Source: CAD feature listing. Evaluate the final solid. Frame: model axes, mm. Face numbers are marked on the shaded views. A direction names the side the tool comes from. Coordinates: 2 decimals unless noted, no trailing zeros. Write each loop counter-clockwise with the first axis right and the second up, starting at its lowest first coordinate (ties: lowest second). Pieces come first, ordered by that corner, then holes. Notation, with made-up numbers: M 71,4 L 100,4 A16 ccw 100,20 Z; hole C -1,0 d11. An arc over 180 degrees is marked long. One line per item, written item: value. Start each with the question number.
Item 1: Cut plane D-D, the plane z = 3.25. State how many separate pieces and enclosed holes the cut face has, then the cut area to 3 significant figures.
Item 2: Pin query (flat end, axial travel): P1, Ø3.5, axis at x = 14, y = 15, coming from the +Z side; P2, Ø2.5, axis at x = -1, z = 3.5, coming from the +Y side. Return the tip coordinate at first contact, or that it passes through.
Item 3: Cut plane A-A, the plane y = -26.5. Output: boundary loops of the cut face in (x, z).
Item 4: Cut plane B-B, the plane x = 10. Output: boundary loops of the cut face in (y, z).
Item 5: Mould query, pull axis X, two halves, no side actions, for the marked faces 1, 2 and 3. Classes: released by +X, released by -X, zero draft, split by the parting line, or undercut.
Item 6: Cut plane C-C, the plane x = -1. Output: boundary loops of the cut face in (y, z), then the cut area to 3 significant figures.
Item 7: Set-up query: the marked faces 4, 5 and 6. Return all of +Z, -Z, +X, -X, +Y, -Y with unobstructed straight access to the full face (end or side cutting, diameter ignored); none if empty.
Item 8: Ray query, L1, parallel to Y at x = 2, z = 2.25; L2, parallel to Y at x = -6, z = 2.1; L3, parallel to X at y = 6, z = 1.6. Return the intervals inside material, ascending. Write a range as from..to.
```python
from build123d import *

# Parameters (mm, degrees)
SKETCH_1_W          = 35
SKETCH_1_H          = 60
EXTRUDE_1_DEPTH     = 5
SKETCH_2_R          = 1.5
SKETCH_2_R_2        = 0.5
SKETCH_2_W          = 15
SKETCH_2_H          = 10
CUT_EXTRUDE_1_DEPTH = 36.089172119
SKETCH_3_R          = 1.5
CUT_EXTRUDE_2_DEPTH = 47.368092477
HOLE_WIZARD_M3_1_D  = 2.5
CHAMFER_1_SIZE      = 0.5


with BuildPart() as part:
    # 草图1 → 凸台-拉伸1 (new body)
    with BuildSketch(Plane.XY):
        Rectangle(SKETCH_1_W, SKETCH_1_H)
    extrude(amount=EXTRUDE_1_DEPTH)

    # 草图2 → 切除-拉伸1 (cut, through all)
    with BuildSketch(Plane.XY.offset(5)):
        with Locations((-14, 0)):
            Circle(SKETCH_2_R)
        with Locations((-14, -15)):
            Circle(SKETCH_2_R)
        with Locations(Location((14, -15, 0), (0, 0, 180))):
            Circle(SKETCH_2_R)
        with Locations(Location((14, 0, 0), (0, 0, 180))):
            Circle(SKETCH_2_R)
        with Locations((-14, -10)):
            Circle(SKETCH_2_R)
        with Locations((-14, -22)):
            Circle(SKETCH_2_R)
        with Locations(Location((14, -22, 0), (0, 0, 180))):
            Circle(SKETCH_2_R)
        with Locations(Location((14, -10, 0), (0, 0, 180))):
            Circle(SKETCH_2_R)
        with Locations(Location((-14, 22, 0), (0, 0, 180))):
            Circle(SKETCH_2_R)
        with Locations((14, 22)):
            Circle(SKETCH_2_R)
        with Locations((14, 10)):
            Circle(SKETCH_2_R)
        with Locations(Location((-14, 10, 0), (0, 0, 180))):
            Circle(SKETCH_2_R)
        with Locations((14, 15)):
            Circle(SKETCH_2_R)
        with Locations(Location((-14, 15, 0), (0, 0, 180))):
            Circle(SKETCH_2_R)
        with Locations((-5, 0)):
            Circle(SKETCH_2_R_2)
        with Locations((5, 0)):
            Circle(SKETCH_2_R_2)
        with Locations((-14, -5)):
            Circle(SKETCH_2_R)
        with Locations(Location((14, -5, 0), (0, 0, 180))):
            Circle(SKETCH_2_R)
        with Locations((14, 5)):
            Circle(SKETCH_2_R)
        with Locations(Location((-14, 5, 0), (0, 0, 180))):
            Circle(SKETCH_2_R)
        with Locations((-5, 17)):
            Circle(SKETCH_2_R_2)
        with Locations((5, 17)):
            Circle(SKETCH_2_R_2)
        with Locations(Location((5, -17, 0), (0, 0, 180))):
            Circle(SKETCH_2_R_2)
        with Locations(Location((-5, -17, 0), (0, 0, 180))):
            Circle(SKETCH_2_R_2)
        with Locations((0, 25)):
            Rectangle(SKETCH_2_W, SKETCH_2_H)
        with Locations((0, -25)):
            Rectangle(SKETCH_2_W, SKETCH_2_H)
        with BuildLine():
            Line((7.5, 11), (7.5, 6))
            ThreePointArc((7.5, 6), (6.621320344, 3.878679656), (4.5, 3))
            Line((4.5, 3), (-4.5, 3))
            ThreePointArc((-4.5, 3), (-6.621320344, 3.878679656), (-7.5, 6))
            Line((-7.5, 6), (-7.5, 11))
            ThreePointArc((-7.5, 11), (-6.621320344, 13.121320344), (-4.5, 14))
            Line((-4.5, 14), (4.5, 14))
            ThreePointArc((4.5, 14), (6.621320344, 13.121320344), (7.5, 11))
        make_face()
        with BuildLine():
            Line((-4.5, -14), (4.5, -14))
            ThreePointArc((4.5, -14), (6.621320344, -13.121320344), (7.5, -11))
            Line((7.5, -11), (7.5, -6))
            ThreePointArc((7.5, -6), (6.621320344, -3.878679656), (4.5, -3))
            Line((4.5, -3), (-4.5, -3))
            ThreePointArc((-4.5, -3), (-6.621320344, -3.878679656), (-7.5, -6))
            Line((-7.5, -6), (-7.5, -11))
            ThreePointArc((-7.5, -11), (-6.621320344, -13.121320344), (-4.5, -14))
        make_face()
    extrude(amount=-CUT_EXTRUDE_1_DEPTH, mode=Mode.SUBTRACT)

    # 草图3 → 切除-拉伸2 (cut, through all)
    with BuildSketch(Plane(origin=(17.5, 0, 0), x_dir=(0, 0, -1), z_dir=(1, 0, 0))):
        with Locations((-2.5, -26.5)):
            Circle(SKETCH_3_R)
        with Locations((-2.5, 26.5)):
            Circle(SKETCH_3_R)
    extrude(amount=-CUT_EXTRUDE_2_DEPTH, mode=Mode.SUBTRACT)

    # M3 螺纹孔1 (through all)
    with Locations(Plane.XY.offset(5)):
        with Locations((-5, 17), (5, 17), (-5, 0), (5, 0), (-5, -17), (5, -17)):
            Hole(HOLE_WIZARD_M3_1_D / 2)

    # 倒角1
    chamfer_1_edges = [part.edges().sort_by_distance(p)[0] for p in [
        (-15.5, -5, 0),
        (-15.5, -5, 5),
        (15.5, -5, 0),
        (15.5, -5, 5),
        (12.5, 5, 0),
        (12.5, 5, 5),
        (-12.5, 5, 0),
        (-12.5, 5, 5),
        (-17.5, -26.5, 4),
        (17.5, -26.5, 4),
        (-17.5, 26.5, 4),
        (17.5, 26.5, 4),
        (6.25, -17, 5),
        (6.25, -17, 0),
        (-3.75, -17, 5),
        (-3.75, -17, 0),
        (6.25, 0, 5),
        (6.25, 0, 0),
        (-3.75, 0, 5),
        (-3.75, 0, 0),
        (6.25, 17, 5),
        (6.25, 17, 0),
        (-3.75, 17, 5),
        (-3.75, 17, 0),
        (-15.5, 0, 0),
        (-15.5, 0, 5),
        (-15.5, -15, 0),
        (-15.5, -15, 5),
        (15.5, -15, 0),
        (15.5, -15, 5),
        (15.5, 0, 0),
        (15.5, 0, 5),
        (-15.5, -10, 0),
        (-15.5, -10, 5),
        (-15.5, -22, 0),
        (-15.5, -22, 5),
        (15.5, -22, 0),
        (15.5, -22, 5),
        (15.5, -10, 0),
        (15.5, -10, 5),
        (-12.5, 22, 0),
        (-12.5, 22, 5),
        (12.5, 22, 0),
        (12.5, 22, 5),
        (12.5, 10, 0),
        (12.5, 10, 5),
        (-12.5, 10, 0),
        (-12.5, 10, 5),
        (12.5, 15, 0),
        (12.5, 15, 5),
        (-12.5, 15, 0),
        (-12.5, 15, 5),
    ]]
    chamfer(chamfer_1_edges, length=CHAMFER_1_SIZE)


solid = part.part
```
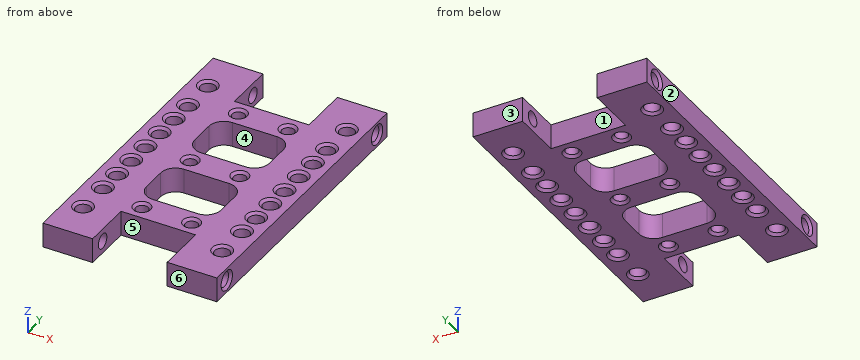
From the geometry:
1. separate pieces: 5
1. enclosed holes: 26
1. area: 1,220 mm²
2. P1: stops at z = 4.75
2. P2: stops at y = 20
3. outline: M -17.5,0 L -7.5,0 L -7.5,1 L -17,1 L -17.5,0.5 Z; M -17.5,4.5 L -17,4 L -7.5,4 L -7.5,5 L -17.5,5 Z; M 7.5,0 L 17.5,0 L 17.5,0.5 L 17,1 L 7.5,1 Z; M 7.5,4 L 17,4 L 17.5,4.5 L 17.5,5 L 7.5,5 Z
4. outline: M -30,0 L 30,0 L 30,5 L -30,5 Z; hole C -26.5,2.5 d3; hole C 26.5,2.5 d3
5. face 1: undercut
5. face 2: released by -X
5. face 3: zero draft
6. outline: M -20,0 L -14,0 L -14,5 L -20,5 Z; M -3,0 L 3,0 L 3,5 L -3,5 Z; M 14,0 L 20,0 L 20,5 L 14,5 Z
6. area: 90.0 mm²
7. face 4: +Z, -Z
7. face 5: +Z, -Z, -Y
7. face 6: +Z, -Z, +X, -X, -Y
8. L1: y = -20..-14, -3..3, 14..20
8. L2: y = -20..-17.75, -16.25..-13.6, -3.4..-0.75, 0.75..3.4, 13.6..16.25, 17.75..20
8. L3: x = -17.5..-15.12, -12.88..-7.5, 7.5..12.88, 15.12..17.5
